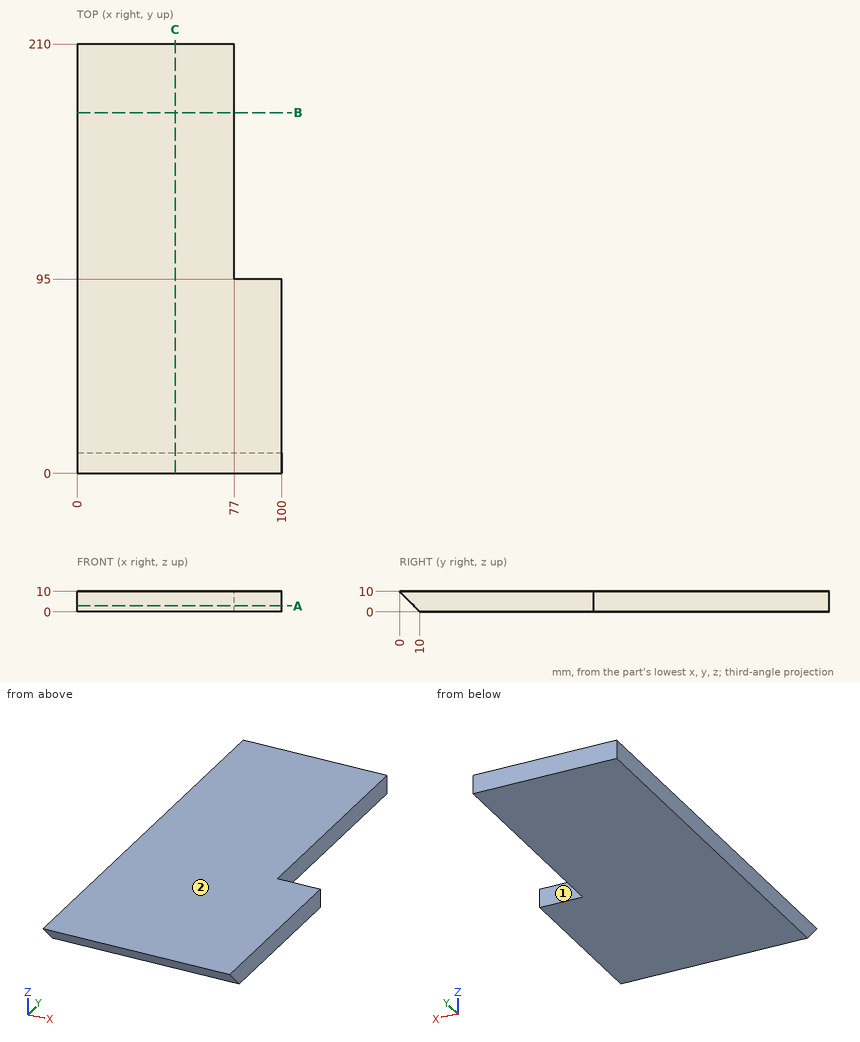
The figure shows three views and two pictorial views of one solid part (mm, origin at its lowest corner). Answer the questions. A direction names the side the tool comes from. Coordinates: 2 decimals unless noted, no trailing zeros. Write each loop counter-clockwise with the first axis right and the second up, starting at its lowest first coordinate (ties: lowest second). Pieces come first, ordered by that corner, then holes. Notation, with made-up numbers: (55, 16.25) -> (91, 16.25) arc R32 cw to (91, 44.25) -> close; hole circle Ø10 at (-4, -27). An arc over 180 degrees is marked (long way). Return JSON: item names as keys, results as strings.
1. A cutting plane is placed at A-A (z = 3). Determine the outline of the cut face in (x, y), and give its area (3 significant figures).
Found:
{"outline": "(0, 7) -> (100, 7) -> (100, 95) -> (77, 95) -> (77, 210) -> (0, 210) -> close", "area": "17,700 mm2"}
2. Each of these flat-tipped pins is pushed along its axis until it touches: P1, Ø6, axis at x = 20.5, z = 9, coming from the -Y side; P2, Ø5, axis at x = 82.5, z = 1.5, coming from the -Y side; P3, Ø1.5, axis at y = 126, z = 6.5, coming from the +X side. Where does it stop, or does it pass through?
Found:
{"P1": "y = 0", "P2": "y = 6", "P3": "x = 77"}
3. Find the intervals of material crossed by line 1 along X through (y, z) = (140.5, 0.75); line 2 along Y through (x, z) = (12, 6); line 3 along Y through (x, z) = (43, 9.5), in increasing order. Write a range as from..to.
Found:
{"line 1": "0..77", "line 2": "4..210", "line 3": "0.5..210"}
4. A tool of negligible diameter and unlimited length cuts with its end or side. For the marked faces 1 and 2, from which of +Z, -Z, +X, -X, +Y, -Y can it reach the whole face along a straight path? Write none if from no direction.
Found:
{"face 1": "+Z, -Z, +X, +Y", "face 2": "+Z, +X, -X, +Y, -Y"}
5. A cutting plane is placed at C-C (x = 48). Determine the outline of the cut face in (y, z), and give its area (3 significant figures).
Found:
{"outline": "(0, 10) -> (10, 0) -> (210, 0) -> (210, 10) -> close", "area": "2,050 mm2"}
6. A cutting plane is placed at B-B (y = 176.5). Determine the outline of the cut face in (x, z).
Found:
{"outline": "(0, 0) -> (77, 0) -> (77, 10) -> (0, 10) -> close"}
